Design review of the part built by this model. Coordinates are the model's own, in mm. Face numbers are marked on the shaded views. A direction names the side the tool comes from. Round coordinates to 2 decimals unless told otherwise and drop trailing zeros. Write each loop counter-clockwise with the first axis right and the second up, starting at its lowest first coordinate (ties: lowest second). Pieces come first, ordered by that corner, then holes. Notation, with made-up numbers: M 30.5,-28 L 56.5,-28 A25 cw 56.5,-6 Z; hole C 57.5,-33 d11. An arc over 180 degrees is marked long. One line per question, with ' | ' between items. Start each with the question number.
Item 1: For L1, parallel to X at y = -28, z = 112.5; L2, parallel to Z at x = -66.75, y = -23.65; L3, parallel to X at y = -26.5, z = 22.5 (3 decimals), list the stretches that pass through material, from the lowest coordinate up.
Item 2: Machinability: for the marked faces 1, 2 and 3, which of the approach directions +Z, -Z, +X, -X, +Y, -Y give a long, thin tool a straight path to every point of the face, cutting with its end or side? Answer none if there is none.
Item 3: Add section B-B, the plane z = 154. State the section outline as (x, y) points (3 decimals), and give its area (3 significant figures).
Item 4: Add section A-A, the plane y = -18.5. State the section outline as (x, z) points (3 decimals).
Item 5: Insertion check: pin 1 Ø17 at (y, z) = (-19, 23.5) entering from +X; pin 2 Ø2 at (y, z) = (-13, 87) entering from -X; pin 3 Ø7.5 at (y, z) = (-20, 142.5) entering from -X. Each pin has a flat end and moves straight along its axis. Give the tip position at first contact, or say it passes through.
```python
from build123d import *

# Parameters (mm, degrees)
F1_DEPTH  = 30
F3_DEPTH  = 20
F5_DEPTH  = 14.986
F6_R      = 10.112
F7_R      = 15.528
F8_R      = 12.7
F10_DEPTH = 23.114
F11_R     = 12.7
F12_R     = 6.35
F13_R     = 4.525
F14_R     = 1.5
F15_DEPTH = 73.613
F16_R     = 1.5
F17_DEPTH = 124.6851495458


with BuildPart() as f1:
    # F0 (on Front) → F1 (new body)
    with BuildSketch(Plane.XZ):
        Polygon((-15.57, 0), (0, 0), (0, 192.28), (-76.2, 192.28), (-76.2, 88.49), (-21.92, 34.21), (-21.92, 22.17), (-15.57, 22.17), align=None)
    extrude(amount=F1_DEPTH)

    # F2 (on face) → F3 (cut)
    with BuildSketch(Plane.XZ.offset(30)):
        Polygon((0, 192.28), (-63.5, 192.28), (-63.5, 93.7505122421), (-9.22, 39.4705122421), (-9.22, 0), (0, 0), align=None)
    extrude(amount=-F3_DEPTH, mode=Mode.SUBTRACT)

    # F4 (on face) → F5 (cut)
    with BuildSketch(Plane.XZ.offset(30)):
        Polygon((-73.612, 192.28), (-76.2, 192.28), (-76.2, 88.49), (-21.92, 34.21), (-21.92, 22.17), (-19.332, 22.17), (-19.332, 35.2819846994), (-73.612, 89.5619846994), align=None)
    extrude(amount=-F5_DEPTH, mode=Mode.SUBTRACT)

    # F6
    f6_edges = [f1.edges().sort_by_distance(p)[0] for p in [
        (-73.612, -22.507, 89.561985),
    ]]
    fillet(f6_edges, radius=F6_R)

    # F7
    f7_edges = [f1.edges().sort_by_distance(p)[0] for p in [
        (-19.332, -22.507, 35.281985),
    ]]
    fillet(f7_edges, radius=F7_R)

    # F8
    f8_edges = [f1.edges().sort_by_distance(p)[0] for p in [
        (-76.2, -7.507, 88.49),
        (-21.92, -7.507, 34.21),
    ]]
    fillet(f8_edges, radius=F8_R)

    # F9 (on face) → F10 (cut)
    with BuildSketch(Plane(origin=(0, 0, 0), x_dir=(1, 0, 0), z_dir=(0, 0, -1))):
        Polygon((-29.2910200357, 0), (0, 0), (0, 3.175), (-14.625, 3.175), (-14.625, 30), (-29.2910200357, 30), align=None)
    extrude(amount=-F10_DEPTH, mode=Mode.SUBTRACT)

    # F11
    f11_edges = [f1.edges().sort_by_distance(p)[0] for p in [
        (-76.2, 0, 143.015256),
        (-75.23327, 0, 88.890433),
        (-49.06, 0, 61.35),
        (-22.88673, 0, 33.809567),
        (-21.92, 0, 26.031744),
    ]]
    fillet(f11_edges, radius=F11_R)

    # F12
    f12_edges = [f1.edges().sort_by_distance(p)[0] for p in [
        (-14.625, -3.175, 11.557),
    ]]
    fillet(f12_edges, radius=F12_R)

    # F13
    f13_edges = [f1.edges().sort_by_distance(p)[0] for p in [
        (-9.22, -10, 19.735256),
        (-36.36, -10, 66.610512),
        (-63.5, -10, 143.015256),
        (-63.5, -20, 93.750512),
        (-9.22, -20, 39.470512),
    ]]
    fillet(f13_edges, radius=F13_R)

    # F14 (on face) → F15 (cut, through all)
    with BuildSketch(Plane(origin=(-73.612, 0, 0), x_dir=(0, -1, 0), z_dir=(-1, 0, 0))):
        with Locations((23.65, 166.88)):
            Circle(F14_R)
        with Locations((23.65, 103.38)):
            Circle(F14_R)
    extrude(amount=-F15_DEPTH, mode=Mode.SUBTRACT)

    # F16 (on face) → F17 (cut, through all)
    with BuildSketch(Plane(origin=(7.9749923497, 0, 7.9749923497), x_dir=(0.7071067812, 0, -0.7071067812), z_dir=(-0.7071067812, 0, -0.7071067812))):
        with Locations((-99.281846784, 23.65)):
            Circle(F16_R)
        with Locations((-61.181846784, 23.65)):
            Circle(F16_R)
    extrude(amount=-F17_DEPTH, mode=Mode.SUBTRACT)


solid = f1.part
```
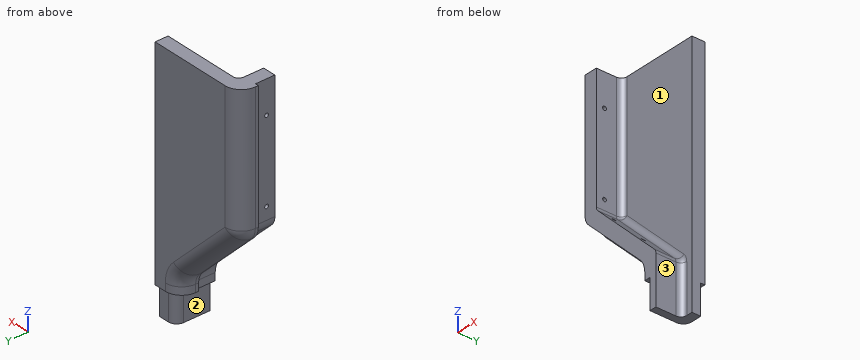
Computed values:
1) L1: x = -73.61 to -63.5 | L2: z = 82.7 to 101.88, 104.88 to 165.38, 168.38 to 192.28 | L3: x = -14.625 to -9.22
2) face 1: +Z, +X, -Y | face 2: -Z, -X, +Y, -Y | face 3: +Z, -Z, +X, -Y
3) outline: M -76.2,-15.014 L -73.612,-15.014 L -73.612,-30 L -63.5,-30 L -63.5,-14.525 A4.525 cw -58.975,-10 L 0,-10 L 0,0 L -63.5,0 A12.7 ccw -76.2,-12.7 Z | area: 947 mm^2
4) outline: M -73.612,93.751 A10.112 ccw -70.65,86.6 L -23.88,39.83 A15.528 cw -19.332,28.85 L -19.332,23.114 L -14.625,23.114 L -14.625,0 L -9.22,0 L -9.22,37.596 A4.525 ccw -10.545,40.796 L -62.175,92.425 A4.525 cw -63.5,95.625 L -63.5,192.28 L -73.612,192.28 Z
5) pin 1: stops at x = -6.76 | pin 2: stops at x = -74.82 | pin 3: stops at x = -73.61
